```python
from build123d import *

# Parameters (mm, degrees)
SKETCH_1_W          = 147
SKETCH_1_H          = 76
EXTRUDE_1_DEPTH     = 12
SKETCH_2_W          = 144
SKETCH_2_H          = 73
CUT_EXTRUDE_1_DEPTH = 10
SKETCH_3_R          = 1.65
CUT_EXTRUDE_2_DEPTH = 166.918654768
CUT_EXTRUDE_3_DEPTH = 10
SKETCH_6_W          = 147
SKETCH_6_H          = 3
CUT_EXTRUDE_4_DEPTH = 166.918654768


with BuildPart() as part:
    # 草图1 → 凸台-拉伸1 (new body)
    with BuildSketch(Plane(origin=(0, 0, 0), x_dir=(1, 0, 0), z_dir=(0, 1, 0))):
        with Locations((73.5, 38)):
            Rectangle(SKETCH_1_W, SKETCH_1_H)
    extrude(amount=EXTRUDE_1_DEPTH)

    # 草图2 → 切除-拉伸1 (cut)
    with BuildSketch(Plane(origin=(0, 12, 0), x_dir=(1, 0, 0), z_dir=(0, 1, 0))):
        with Locations((73.5, 38)):
            Rectangle(SKETCH_2_W, SKETCH_2_H)
    extrude(amount=-CUT_EXTRUDE_1_DEPTH, mode=Mode.SUBTRACT)

    # 草图3 → 切除-拉伸2 (cut, through all)
    with BuildSketch(Plane(origin=(0, 0, -76), x_dir=(-1, 0, 0), z_dir=(0, 0, -1))):
        with Locations((-113.5, 6)):
            Circle(SKETCH_3_R)
        with Locations((-33.5, 6)):
            Circle(SKETCH_3_R)
    extrude(amount=-CUT_EXTRUDE_2_DEPTH, mode=Mode.SUBTRACT)

    # 草图5 → 切除-拉伸3 (cut)
    with BuildSketch(Plane.XZ):
        with BuildLine():
            Line((61.375644347, -46.748711306), (47.375644347, -22.5))
            ThreePointArc((47.375644347, -22.5), (47.375644347, -8.5), (59.5, -1.5))
            Line((59.5, -1.5), (87.5, -1.5))
            ThreePointArc((87.5, -1.5), (99.624355653, -8.5), (99.624355653, -22.5))
            Line((99.624355653, -22.5), (85.624355653, -46.748711306))
            ThreePointArc((85.624355653, -46.748711306), (73.5, -53.748711306), (61.375644347, -46.748711306))
        make_face()
    extrude(amount=-CUT_EXTRUDE_3_DEPTH, mode=Mode.SUBTRACT)

    # 草图6 → 切除-拉伸4 (cut, through all)
    with BuildSketch(Plane(origin=(0, 12, 0), x_dir=(1, 0, 0), z_dir=(0, 1, 0))):
        with Locations((73.5, 74.5)):
            Rectangle(SKETCH_6_W, SKETCH_6_H)
    extrude(amount=-CUT_EXTRUDE_4_DEPTH, mode=Mode.SUBTRACT)


solid = part.part
```
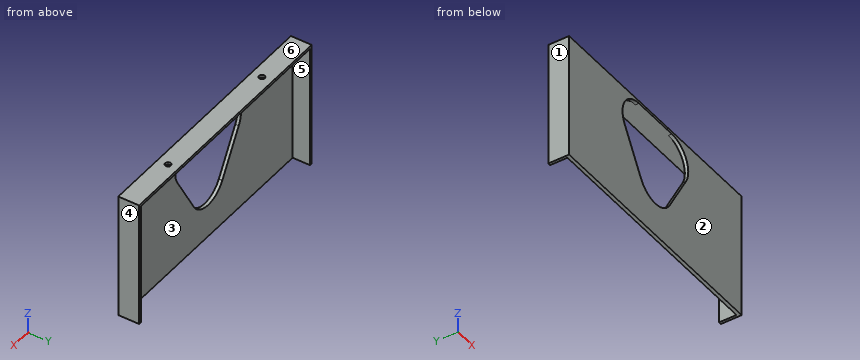
Input: part model. Units: mm. Frame: model coordinates. Face numbers are marked on the shaded views. A direction names the side the tool comes from. Coordinates: 2 decimals unless noted, no trailing zeros. Write each loop counter-clockwise with the first axis right and the second up, starting at its lowest first coordinate (ties: lowest second). Pieces come first, ordered by that corner, then holes.
1) Section A-A on y = 6. Output: boundary loops of the cut face in (x, z).
2) Set-up query: the marked faces 5 and 6. Return all of +Z, -Z, +X, -X, +Y, -Y with unobstructed straight access to the full face (end or side cutting, diameter ignored); none if empty.
3) Section C-C on z = -57. Output: boundary loops of the cut face in (x, y).
4) Pin query (flat end, axial travel): pin 1 Ø1 at (x, z) = (102, -65) entering from +Y; pin 2 Ø5.5 at (x, y) = (113.5, 6) entering from -Z. Return the tip coordinate at first contact, or that it passes through.
5) Section B-B on x = 33.5. Output: boundary loops of the cut face in (y, z).
6) Section D-D on z = -20. Output: boundary loops of the cut face in (x, y).
7) Mould query, pull axis X, two halves, no side actions, for the marked faces 1, 2, 3 and 4. Classes: pulls with the +X half, pulls with the -X half, needs draft (parallel to the pull), parting line crosses it, or undercut.
8) Material intervals for line 1 along X through (y, z) = (9.75, -63.5); line 2 along Z through (x, y) = (59, 7); line 3 along Y through (x, z) = (33.5, -1.2), sorted ascending.
Check result:
1. outline: (0, -73) - (1.5, -73) - (1.5, -1.5) - (31.85, -1.5) - (31.85, 0) - (0, 0) - close; (35.15, -1.5) - (111.85, -1.5) - (111.85, 0) - (35.15, 0) - close; (115.15, -1.5) - (145.5, -1.5) - (145.5, -73) - (147, -73) - (147, 0) - (115.15, 0) - close
2. face 5: -Z, +Y
2. face 6: +Z, +X, -X, +Y, -Y
3. outline: (0, 0) - (147, 0) - (147, 12) - (145.5, 12) - (145.5, 2) - (1.5, 2) - (1.5, 12) - (0, 12) - close
4. pin 1: stops at y = 2
4. pin 2: stops at z = -1.5
5. outline: (0, -73) - (2, -73) - (2, -1.5) - (4.35, -1.5) - (4.35, 0) - (0, 0) - close; (7.65, -1.5) - (12, -1.5) - (12, 0) - (7.65, 0) - close
6. outline: (0, 0) - (46.24, 0) - (46.24, 2) - (1.5, 2) - (1.5, 12) - (0, 12) - close; (100.76, 0) - (147, 0) - (147, 12) - (145.5, 12) - (145.5, 2) - (100.76, 2) - close
7. face 1: pulls with the -X half
7. face 2: needs draft
7. face 3: undercut
7. face 4: pulls with the +X half
8. line 1: x = 0 to 1.5, 145.5 to 147
8. line 2: z = -1.5 to 0
8. line 3: y = 0 to 4.35, 7.65 to 12
